Geometry: final body of the model. Coordinates: model frame, mm. A direction names the side the tool comes from. Round coordinates to 2 decimals unless told otherwise and drop trailing zeros. Loops run counter-clockwise (first coordinate to the right, second up) from the corner with the lowest first, then second, coordinate; pieces in that order, holes last. Notation, with made-up numbers: M 72,51 L 100,51 A21 cw 100,88 Z; hole C 36,59 d3. An arc over 180 degrees is marked long. Return JSON: item names as keys, results as strings.
from build123d import *

# Parameters (mm, degrees)
SKETCH2_W           = 32
SKETCH2_H           = 70
BOSS_EXTRUDE1_DEPTH = 2
BOSS_EXTRUDE2_DEPTH = 2
BOSS_EXTRUDE3_DEPTH = 2
SKETCH6_W           = 28
SKETCH6_H           = 30
BOSS_EXTRUDE4_DEPTH = 2
FILLET1_R           = 1
FILLET2_R           = 1
FILLET3_R           = 1
FILLET4_R           = 1
FILLET5_R           = 1
SKETCH7_W           = 28
SKETCH7_H           = 36.055512754
SKETCH7_W_2         = 27
SKETCH7_H_2         = 27
BOSS_EXTRUDE5_DEPTH = 2


with BuildPart() as part:
    # Sketch2 → Boss-Extrude1 (new body)
    with BuildSketch(Plane(origin=(0, 0, 0), x_dir=(1, 0, 0), z_dir=(0, 1, 0))):
        Rectangle(SKETCH2_W, SKETCH2_H)
    extrude(amount=BOSS_EXTRUDE1_DEPTH)



with BuildPart() as body_2:
    # Sketch4 → Boss-Extrude2 (new body)
    with BuildSketch(Plane.ZY.offset(16)):
        Polygon((35, 2), (15, 32), (-35, 32), (-35, 2), align=None)
    extrude(amount=-BOSS_EXTRUDE2_DEPTH)


with BuildPart() as body_3:
    # Sketch5 → Boss-Extrude3 (new body)
    with BuildSketch(Plane(origin=(16, 0, 0), x_dir=(0, 0, -1), z_dir=(1, 0, 0))):
        Polygon((-35, 2), (-15, 32), (35, 32), (35, 2), align=None)
    extrude(amount=-BOSS_EXTRUDE3_DEPTH)


with BuildPart() as part_1:
    add(part.part)

    add(body_2.part)  # Boss-Extrude4 merges body 2

    add(body_3.part)  # Boss-Extrude4 merges body 3
    # Sketch6 → Boss-Extrude4 (add)
    with BuildSketch(Plane(origin=(0, 0, -35), x_dir=(-1, 0, 0), z_dir=(0, 0, -1))):
        with Locations((0, 17)):
            Rectangle(SKETCH6_W, SKETCH6_H)
    extrude(amount=-BOSS_EXTRUDE4_DEPTH)

    # Fillet1
    fillet1_edges = [part_1.edges().sort_by_distance(p)[0] for p in [
        (16, 32, -10),
    ]]
    fillet(fillet1_edges, radius=FILLET1_R)

    # Fillet2
    fillet2_edges = [part_1.edges().sort_by_distance(p)[0] for p in [
        (-16, 32, -10),
    ]]
    fillet(fillet2_edges, radius=FILLET2_R)

    # Fillet3
    fillet3_edges = [part_1.edges().sort_by_distance(p)[0] for p in [
        (0, 32, -35),
        (16, 15.5, -35),
        (15.707106781, 31.707106781, -35),
        (-16, 15.5, -35),
        (-15.707106781, 31.707106781, -35),
    ]]
    fillet(fillet3_edges, radius=FILLET3_R)

    # Fillet4
    fillet4_edges = [part_1.edges().sort_by_distance(p)[0] for p in [
        (0, 0, -35),
        (16, 0, 0.5),
        (-16, 0, 0.5),
        (-15.707106781, 0, -34.707106781),
        (15.707106781, 0, -34.707106781),
    ]]
    fillet(fillet4_edges, radius=FILLET4_R)

    # Fillet5
    fillet5_edges = [part_1.edges().sort_by_distance(p)[0] for p in [
        (16, 1.5, 35),
        (-16, 1.5, 35),
        (0, 0, 35),
        (15.707106781, 0.292893219, 35),
        (-15.707106781, 0.292893219, 35),
    ]]
    fillet(fillet5_edges, radius=FILLET5_R)

    # Sketch7 → Boss-Extrude5 (add)
    with BuildSketch(Plane(origin=(0, 16.769230769, 25.153846154), x_dir=(1, 0, 0), z_dir=(0, 0.5547001962252296, 0.8320502943378435))):
        with Locations((0, 0.277350098)):
            Rectangle(SKETCH7_W, SKETCH7_H)
        Rectangle(SKETCH7_W_2, SKETCH7_H_2, mode=Mode.SUBTRACT)
    extrude(amount=-BOSS_EXTRUDE5_DEPTH)


solid = part_1.part
Q1. Section query B-B (z = -18.5). Output: boundary loops of the cut face in (x, y), plus the area to 3 significant figures.
Determined:
{"outline": "M -16,1 A1 ccw -15,0 L 15,0 A1 ccw 16,1 L 16,31 A1 ccw 15,32 L 14,32 L 14,2 L -14,2 L -14,32 L -15,32 A1 ccw -16,31 Z", "area": "183 mm^2"}
Q2. Material intervals for L1, parallel to X at y = 4, z = -2; L2, parallel to X at y = 19.5, z = 21; L3, parallel to Y at x = -5, z = -11, sorted ascending.
Determined:
{"L1": "x = -16 to -14, 14 to 16", "L2": "x = -16 to -13.5, 13.5 to 16", "L3": "y = 0 to 2"}
Q3. Section query C-C (y = 25). Output: boundary loops of the cut face in (x, z), plus the area to 3 significant figures.
Determined:
{"outline": "M -16,-34 A1 ccw -15,-35 L 15,-35 A1 ccw 16,-34 L 16,19.67 L 13.5,19.67 L 13.5,17.26 L 14,17.26 L 14,-33 L -14,-33 L -14,17.26 L -13.5,17.26 L -13.5,19.67 L -16,19.67 Z", "area": "277 mm^2"}
Q4. Section query A-A (x = -3.5). Output: boundary loops of the cut face in (y, z), plus the area to 3 significant figures.
Determined:
{"outline": "M 0,-34 A1 ccw 1,-35 L 31,-35 A1 ccw 32,-34 L 32,-33 L 2,-33 L 2,32.6 L 4.43,30.98 L 5.54,32.64 L 2,35 L 1,35 A1 ccw 0,34 Z; M 26.89,16 L 30.89,13.34 L 32,15 L 28,17.67 Z", "area": "216 mm^2"}
Q5. Section query D-D (y = 14.5). Output: boundary loops of the cut face in (x, z), plus the area to 3 significant figures.
Determined:
{"outline": "M -16,-34 A1 ccw -15,-35 L 15,-35 A1 ccw 16,-34 L 16,26.67 L 13.5,26.67 L 13.5,24.26 L 14,24.26 L 14,-33 L -14,-33 L -14,24.26 L -13.5,24.26 L -13.5,26.67 L -16,26.67 Z", "area": "305 mm^2"}
Q6. Reachability of faces 1 (the flat face through (14.5, 32, -16.9)), 2 (the flat face through (-2.14, 27.21, 15.79)), 3 (the flat face through (-0.19, 4.99, 31.82)), 4 (the flat face through (-0.19, 27.45, 16.84)) from +Z, -Z, +X, -X, +Y, -Y: full face, straight path, thin tool, end or side. Return the list, or none.
Determined:
{"face 1": "+Z, -Z, +X, -X, +Y", "face 2": "none", "face 3": "+Y", "face 4": "+Z"}
Q7. Pin query (flat end, axial travel): pin 1 (8.5 mm diameter, centred on x = 1.5, y = 12.5, fed in from +Z); pin 2 (5 mm diameter, centred on x = 6.5, z = 18.5, fed in from +Y); pin 3 (6 mm diameter, centred on x = -7.5, z = -18.5, fed in from +Y). Return the tip coordinate at first contact, or that it passes through.
Determined:
{"pin 1": "stops at z = -33", "pin 2": "stops at y = 30.5", "pin 3": "stops at y = 2"}
Q8. Pull-direction query (X, two-part tool) for faces 5 (the flat face through (-16, 16, 0)), 6 (the flat face through (0, 16, -35)), 7 (the flat face through (0, 17, -33)); classes: pulls with the +X half, pulls with the -X half, needs draft (parallel to the pull), parting line crosses it, or undercut.
Determined:
{"face 5": "pulls with the -X half", "face 6": "needs draft", "face 7": "undercut"}
